```python
from build123d import *

# Parameters (mm, degrees)
SKETCH1_W           = 14.7
SKETCH1_H           = 3
SKETCH1_W_2         = 3
SKETCH1_H_2         = 14.7
BOSS_EXTRUDE1_DEPTH = 3
FILLET1_R           = 5


with BuildPart() as part:
    # Sketch1 → Boss-Extrude1 (new body)
    with BuildSketch(Plane.XY):
        Polygon((33.892723269, -30.02061011), (12.617997994, -7.295335385), (-10.107276731, -30.02061011), (7.542723269, -30.02061011), (22.242723269, -30.02061011), align=None)
        with Locations((14.892723269, -31.52061011)):
            Rectangle(SKETCH1_W, SKETCH1_H)
        Polygon((12.617997994, -7.295335385), (-10.107276731, 16.97938989), (-10.107276731, 2.32938989), (-10.107276731, -12.37061011), (-10.107276731, -30.02061011), align=None)
        with Locations((-11.607276731, -5.02061011)):
            Rectangle(SKETCH1_W_2, SKETCH1_H_2)
    extrude(amount=BOSS_EXTRUDE1_DEPTH)

    # Fillet1
    fillet1_edges = [part.edges().sort_by_distance(p)[0] for p in [
        (33.892723269, -30.02061011, 1.5),
        (-10.107276731, 16.97938989, 1.5),
    ]]
    fillet(fillet1_edges, radius=FILLET1_R)


solid = part.part
```
Geometry: final body of the model. Coordinates: model frame, mm. A direction names the side the tool comes from. Give positions to 0.01 mm unless a question says otherwise; leave off trailing zeros. Loops run counter-clockwise (first coordinate to the right, second up) from the corner with the lowest first, then second, coordinate; pieces in that order, holes last. Notation, with made-up numbers: (84, 66) - (90, 66) arc R17 cw to (90, 73) - close; hole circle Ø10 at (32.25, -26.75). An arc over 180 degrees is marked (long way). Answer as CSV lines item,"result". Start each with the question number.
(1) Section query A-A (z = 2.55). Output: boundary loops of the cut face in (x, y).
(2) Reachability of faces 1 (the face through (-10.107, 3, 1)), 2 (the face through (15, -33.021, 1)), 3 (the face through (22.243, -32, 1)), 4 (the face through (-1, -30.021, 1)) from +Z, -Z, +X, -X, +Y, -Y: full face, straight path, thin tool, end or side. Return the list, or none.
(3) Section query B-B (x = 3.5). Output: boundary loops of the cut face in (y, z).
(4) Section query C-C (y = -5.5). Output: boundary loops of the cut face in (x, z), and give its area (3 significant figures).
(5) Ray query, line 1 along Y through (x, z) = (1, 1.9); line 2 along X through (y, z) = (-29, 2.05); line 3 along Y through (x, z) = (8, 0.6). Return the intervals inside material, ascending. Write a range as [from, to].
(6) Pin query (flat end, axial travel): P1, Ø1, axis at y = 3.5, z = 1.5, coming from the -X side; P2, Ø0.9, axis at y = -32, z = 1.5, coming from the -X side; P3, Ø1, axis at y = 5, z = 0.5, coming from the +X side; P4, Ø10, axis at x = 23, y = -5.5, coming from the +Z side. Return the tip coordinate at first contact, or that it passes through.
Worked answers:
1,outline,"(-13.11, -12.37) - (-10.11, -12.37) - (-10.11, -30.02) - (7.54, -30.02) - (7.54, -33.02) - (22.24, -33.02) - (22.24, -30.02) - (22.36, -30.02) arc R5 ccw to (26.01, -21.6) - (-1.46, 7.74) arc R5 ccw to (-10.11, 4.32) - (-10.11, 2.33) - (-13.11, 2.33) - close"
2,face 1,"+Z, -Z, -X, +Y"
2,face 2,"+Z, -Z, +X, -X, -Y"
2,face 3,"+Z, -Z, +X, -Y"
2,face 4,"+Z, -Z, -X, -Y"
3,outline,"(-30.02, 0) - (2.44, 0) - (2.44, 3) - (-30.02, 3) - close"
4,outline,"(-13.11, 0) - (10.94, 0) - (10.94, 3) - (-13.11, 3) - close"
4,area,"72.1 mm^2"
5,line 1,"y = [-30.02, 5.11]"
5,line 2,"x = [-10.11, 25.39]"
5,line 3,"y = [-33.02, -2.36]"
6,P1,"stops at x = -10.11"
6,P2,"stops at x = 7.54"
6,P3,"stops at x = 1.58"
6,P4,"passes through"
